Source: CAD feature listing. Evaluate the final solid. Frame: model axes, mm. A direction names the side the tool comes from. Give positions to 0.01 mm unless a question says otherwise; leave off trailing zeros. Answer in a Markdown table with one row per item.
```python
from build123d import *

# Parameters (mm, degrees)
SKETCH1_R            = 150
BOSS_EXTRUDE3_DEPTH  = 10
CUT_EXTRUDE2_DEPTH   = 10
BOSS_EXTRUDE4_DEPTH  = 1.8
SKETCH6_W            = 3
SKETCH6_H            = 7
BOSS_EXTRUDE5_DEPTH  = 2
SKETCH7_W            = 7
SKETCH7_H            = 3
BOSS_EXTRUDE6_DEPTH  = 2
SKETCH8_W            = 10
SKETCH8_H            = 10
CUT_EXTRUDE3_DEPTH   = 5
SKETCH9_W            = 9.193751657
SKETCH9_H            = 8.277315045
BOSS_EXTRUDE7_DEPTH  = 4.35
CHAMFER1_SIZE        = 1
CUT_EXTRUDE4_DEPTH   = 1.7
CUT_EXTRUDE5_DEPTH   = 0.8
FILLET1_R            = 3
FILLET2_R            = 1.4
SKETCH12_W           = 10.671911796
SKETCH12_H           = 9.690192172
CUT_EXTRUDE6_DEPTH   = 11
SKETCH13_W           = 9.731136712
SKETCH13_H           = 8.6
BOSS_EXTRUDE8_DEPTH  = 10
SKETCH14_W           = 9.731136712
SKETCH14_H           = 8.6
CUT_EXTRUDE7_DEPTH   = 5
FILLET3_R            = 1
FILLET4_R            = 1.2
CUT_EXTRUDE8_DEPTH   = 3.5
FILLET5_R            = 2.5
FILLET6_R            = 9
SKETCH16_W           = 0.25
SKETCH16_H           = 5
BOSS_EXTRUDE9_DEPTH  = 11.5
SKETCH17_W           = 9.5
SKETCH17_H           = 5
BOSS_EXTRUDE12_DEPTH = 0.13
SKETCH19_W           = 9.5
SKETCH19_H           = 5
BOSS_EXTRUDE13_DEPTH = 0.85
CHAMFER2_SIZE        = 1


with BuildPart() as part:
    # Sketch1 → Boss-Extrude3 (new body)
    with BuildSketch(Plane(origin=(0, 0, 0), x_dir=(1, 0, 0), z_dir=(0, 1, 0))):
        with Locations(Location((0, 0, 0), (0, 0, 270))):
            Circle(SKETCH1_R)
    extrude(amount=BOSS_EXTRUDE3_DEPTH)

    # Sketch4 → Cut-Extrude2 (cut)
    with BuildSketch(Plane(origin=(0, 10, 0), x_dir=(1, 0, 0), z_dir=(0, 1, 0))):
        Polygon((0, 0), (0, 162.329653064), (183.678217859, 162.329653064), (183.678217859, -176.427761891), (-217.916482153, -176.427761891), (-217.916482153, 0), align=None)
    extrude(amount=-CUT_EXTRUDE2_DEPTH, mode=Mode.SUBTRACT)

    # Sketch5 → Boss-Extrude4 (add)
    with BuildSketch(Plane(origin=(0, 10, 0), x_dir=(1, 0, 0), z_dir=(0, 1, 0))):
        with BuildLine():
            Line((0, 3.825), (0, 0))
            Line((0, 0), (-3.825, 0))
            ThreePointArc((-3.825, 0), (-2.704683438, 2.704683438), (0, 3.825))
        make_face()
    extrude(amount=BOSS_EXTRUDE4_DEPTH)

    # Sketch6 → Boss-Extrude5 (add)
    with BuildSketch(Plane(origin=(0, 10, 0), x_dir=(1, 0, 0), z_dir=(0, 1, 0))):
        with Locations((-28.5, 3.5)):
            Rectangle(SKETCH6_W, SKETCH6_H)
    extrude(amount=BOSS_EXTRUDE5_DEPTH)

    # Sketch7 → Boss-Extrude6 (add)
    with BuildSketch(Plane(origin=(0, 10, 0), x_dir=(1, 0, 0), z_dir=(0, 1, 0))):
        with Locations((-3.5, 28.5)):
            Rectangle(SKETCH7_W, SKETCH7_H)
    extrude(amount=BOSS_EXTRUDE6_DEPTH)

    # Sketch8 → Cut-Extrude3 (cut)
    with BuildSketch(Plane(origin=(0, 10, 0), x_dir=(1, 0, 0), z_dir=(0, 1, 0))):
        with Locations((-95, 5)):
            Rectangle(SKETCH8_W, SKETCH8_H)
    extrude(amount=-CUT_EXTRUDE3_DEPTH, mode=Mode.SUBTRACT)

    # Sketch9 → Boss-Extrude7 (add)
    with BuildSketch(Plane(origin=(0, 10, 0), x_dir=(1, 0, 0), z_dir=(0, 1, 0))):
        with Locations((4.596875828, 95.138657523)):
            Rectangle(SKETCH9_W, SKETCH9_H)
    extrude(amount=-BOSS_EXTRUDE7_DEPTH)

    # Chamfer1
    chamfer1_edges = [part.edges().sort_by_distance(p)[0] for p in [
        (9.193751657, 7.825, -99.277315045),
        (9.193751657, 7.825, -91),
    ]]
    chamfer(chamfer1_edges, length=CHAMFER1_SIZE)

    # Sketch10 → Cut-Extrude4 (cut)
    with BuildSketch(Plane.XZ):
        with BuildLine():
            Line((-140.926536809, 0), (-144.178447036, 0))
            ThreePointArc((-144.178447036, 0), (-101.9495576, -101.9495576), (0, -144.178447036))
            Line((0, -144.178447036), (0, -140.926536809))
            ThreePointArc((0, -140.926536809), (-99.650109827, -99.650109827), (-140.926536809, 0))
        make_face()
    extrude(amount=-CUT_EXTRUDE4_DEPTH, mode=Mode.SUBTRACT)

    # Sketch11 → Cut-Extrude5 (cut)
    with BuildSketch(Plane(origin=(0, 0, 0), x_dir=(-1, 0, 0), z_dir=(0, -1, 0))):
        Polygon((47, 0), (50, 0), (50, 50), (0, 50), (0, 47), (47, 47), align=None)
    extrude(amount=-CUT_EXTRUDE5_DEPTH, mode=Mode.SUBTRACT)

    # Fillet1
    fillet1_edges = [part.edges().sort_by_distance(p)[0] for p in [
        (-106.066017178, 0, -106.066017178),
    ]]
    fillet(fillet1_edges, radius=FILLET1_R)

    # Fillet2
    fillet2_edges = [part.edges().sort_by_distance(p)[0] for p in [
        (0, 5.65, -95.138657523),
    ]]
    fillet(fillet2_edges, radius=FILLET2_R)

    # Sketch12 → Cut-Extrude6 (cut)
    with BuildSketch(Plane(origin=(0, 0, 0), x_dir=(-1, 0, 0), z_dir=(0, -1, 0))):
        with Locations((-5.335955898, 95.265421493)):
            Rectangle(SKETCH12_W, SKETCH12_H)
    extrude(amount=-CUT_EXTRUDE6_DEPTH, mode=Mode.SUBTRACT)

    # Sketch13 → Boss-Extrude8 (add)
    with BuildSketch(Plane(origin=(0, 0, 0), x_dir=(-1, 0, 0), z_dir=(0, -1, 0))):
        with Locations((-4.865568356, 95.8)):
            Rectangle(SKETCH13_W, SKETCH13_H)
    extrude(amount=-BOSS_EXTRUDE8_DEPTH)

    # Sketch14 → Cut-Extrude7 (cut)
    with BuildSketch(Plane(origin=(0, 0, 0), x_dir=(-1, 0, 0), z_dir=(0, -1, 0))):
        with Locations((-4.865568356, 95.8)):
            Rectangle(SKETCH14_W, SKETCH14_H)
    extrude(amount=-CUT_EXTRUDE7_DEPTH, mode=Mode.SUBTRACT)

    # Fillet3
    fillet3_edges = [part.edges().sort_by_distance(p)[0] for p in [
        (0, 5, -95.8),
    ]]
    fillet(fillet3_edges, radius=FILLET3_R)

    # Fillet4
    fillet4_edges = [part.edges().sort_by_distance(p)[0] for p in [
        (9.731136712, 7.5, -91.5),
        (9.731136712, 7.5, -100.1),
    ]]
    fillet(fillet4_edges, radius=FILLET4_R)

    # Sketch15 → Cut-Extrude8 (cut)
    with BuildSketch(Plane(origin=(0, 10, 0), x_dir=(1, 0, 0), z_dir=(0, 1, 0))):
        with BuildLine():
            Line((-84.010224854, 7.071067812), (-84.010224854, 17.341351392))
            Line((-84.010224854, 17.341351392), (-106.385767568, 17.341351392))
            Line((-106.385767568, 17.341351392), (-106.385767568, 7.071067812))
            Line((-106.385767568, 7.071067812), (-139.141411083, 7.071067812))
            ThreePointArc((-139.141411083, 7.071067812), (-98.514801625, 98.514801625), (-7.071067812, 139.141411083))
            Line((-7.071067812, 139.141411083), (-7.071067812, 59.581876439))
            ThreePointArc((-7.071067812, 59.581876439), (-42.426406871, 42.426406871), (-59.581876439, 7.071067812))
            Line((-59.581876439, 7.071067812), (-84.010224854, 7.071067812))
        make_face()
    extrude(amount=-CUT_EXTRUDE8_DEPTH, mode=Mode.SUBTRACT)

    # Fillet5
    fillet5_edges = [part.edges().sort_by_distance(p)[0] for p in [
        (-84.010224854, 8.25, -17.341351392),
        (-106.385767568, 8.25, -17.341351392),
    ]]
    fillet(fillet5_edges, radius=FILLET5_R)

    # Fillet6
    # the kernel refuses this fillet: 9 mm, written as the material it adds along each edge
    with BuildSketch(Plane(origin=(-103.885767568, 6.5, -14.841351392), x_dir=(-1, 0, 0), z_dir=(0, 0, 1))) as fillet6_piece_1:
        with BuildLine():
            CenterArc((9.623903424, -9), FILLET6_R, 90, 52.330113036)
            Line((9.623903424, 0), (2.5, 0))
            Line((2.5, 0), (2.5, -3.5))
        make_face()
    revolve(axis=Axis((-103.885767568, 6.5, -14.841351392), (0, -1, 0)), revolution_arc=90)
    with BuildSketch(Plane(origin=(-86.510224854, 6.5, -14.841351392), x_dir=(0, 0, -1), z_dir=(-1, 0, 0))) as fillet6_piece_2:
        with BuildLine():
            CenterArc((9.623903424, -9), FILLET6_R, 90, 52.330113036)
            Line((9.623903424, 0), (2.5, 0))
            Line((2.5, 0), (2.5, -3.5))
        make_face()
    revolve(axis=Axis((-86.510224854, 6.5, -14.841351392), (0, -1, 0)), revolution_arc=90)
    with BuildSketch(Plane(origin=(0, 6.5, 0), x_dir=(-0.9970291212395074, 0, 0.07702552434340171), z_dir=(0.07702552434340171, 0, 0.9970291212395074))) as fillet6_piece_3_section:
        with BuildLine():
            CenterArc((132.197065128, -9), FILLET6_R, 37.669886964, 52.330113036)
            Line((132.197065128, 0), (139.320968552, 0))
            Line((139.320968552, 0), (139.320968552, -3.5))
        make_face()
    fillet6_piece_3 = revolve(axis=Axis((0, 6.5, 0), (0, -1, 0)), revolution_arc=98.835226115, mode=Mode.PRIVATE)
    fillet6_piece_3 = split(fillet6_piece_3, bisect_by=Plane(origin=(0, 6.5, 0), z_dir=(-1, 0, 0)), keep=Keep.TOP, mode=Mode.PRIVATE)
    fillet6_piece_3 = split(fillet6_piece_3, bisect_by=Plane(origin=(0, 6.5, 0), z_dir=(0, 0, -1)), keep=Keep.TOP, mode=Mode.PRIVATE)
    add(fillet6_piece_3)
    with BuildSketch(Plane(origin=(-88.576009007, 6.5, -7.071067812), x_dir=(0, 1, 0), z_dir=(-1, 0, 0))) as fillet6_piece_4_section:
        with BuildLine():
            CenterArc((9, 7.123903424), FILLET6_R, 180, 52.330113036)
            Line((0, 7.123903424), (0, 0))
            Line((0, 0), (3.5, 0))
        make_face()
    fillet6_piece_4 = extrude(amount=68.375160637, mode=Mode.PRIVATE)
    fillet6_piece_4 = fillet6_piece_4 & Plane(origin=(0, 6.5, 0), x_dir=(0, 0, 1), z_dir=(0, -1, 0)) * Cylinder(150, 166, mode=Mode.PRIVATE)
    fillet6_piece_4 = split(fillet6_piece_4, bisect_by=Plane(origin=(-100, 6.5, -7.071067812), z_dir=(-1, 0, 0)), keep=Keep.TOP, mode=Mode.PRIVATE)
    add(fillet6_piece_4)
    with BuildSketch(Plane(origin=(-86.510224854, 6.5, -17.341351392), x_dir=(0, 1, 0), z_dir=(-1, 0, 0))) as fillet6_piece_5:
        with BuildLine():
            CenterArc((9, 7.123903424), FILLET6_R, 180, 52.330113036)
            Line((0, 7.123903424), (0, 0))
            Line((0, 0), (3.5, 0))
        make_face()
    extrude(amount=17.375542715)
    with BuildSketch(Plane(origin=(-41.772117878, 6.5, -7.071067812), x_dir=(0, 1, 0), z_dir=(-1, 0, 0))) as fillet6_piece_6_section:
        with BuildLine():
            CenterArc((9, 7.123903424), FILLET6_R, 180, 52.330113036)
            Line((0, 7.123903424), (0, 0))
            Line((0, 0), (3.5, 0))
        make_face()
    fillet6_piece_6 = extrude(amount=60.047865536, mode=Mode.PRIVATE)
    fillet6_piece_6 = split(fillet6_piece_6, bisect_by=Plane(origin=(-90, 6.5, -7.071067812), z_dir=(1, 0, 0)), keep=Keep.TOP, mode=Mode.PRIVATE)
    add(fillet6_piece_6)
    with BuildSketch(Plane(origin=(-7.071067812, 6.5, -156.951169644), x_dir=(0, 1, 0), z_dir=(0, 0, 1))) as fillet6_piece_7_section:
        with BuildLine():
            CenterArc((9, 7.123903424), FILLET6_R, 180, 52.330113036)
            Line((0, 7.123903424), (0, 0))
            Line((0, 0), (3.5, 0))
        make_face()
    fillet6_piece_7 = extrude(amount=115.179051766, mode=Mode.PRIVATE)
    fillet6_piece_7 = fillet6_piece_7 & Plane(origin=(0, 6.5, 0), x_dir=(0, 0, 1), z_dir=(0, -1, 0)) * Cylinder(150, 259, mode=Mode.PRIVATE)
    add(fillet6_piece_7)
    with BuildSketch(Plane(origin=(0, 6.5, 0), x_dir=(0.17783871438849583, 0, -0.9840596484282074), z_dir=(0.9840596484282074, 0, 0.17783871438849583))) as fillet6_piece_8_section:
        with BuildLine():
            CenterArc((67.123903424, 9), FILLET6_R, 217.669886964, 52.330113036)
            Line((67.123903424, 0), (60, 0))
            Line((60, 0), (60, 3.5))
        make_face()
    fillet6_piece_8 = revolve(axis=Axis((0, 6.5, 0), (0, 1, 0)), revolution_arc=110.487792536, mode=Mode.PRIVATE)
    fillet6_piece_8 = split(fillet6_piece_8, bisect_by=Plane(origin=(0, 6.5, 0), z_dir=(-1, 0, 0)), keep=Keep.TOP, mode=Mode.PRIVATE)
    fillet6_piece_8 = split(fillet6_piece_8, bisect_by=Plane(origin=(0, 6.5, 0), z_dir=(0, 0, -1)), keep=Keep.TOP, mode=Mode.PRIVATE)
    add(fillet6_piece_8)
    with BuildSketch(Plane(origin=(-84.010224854, 6.5, 10.738690749), x_dir=(0, 1, 0), z_dir=(0, 0, -1))) as fillet6_piece_9_section:
        with BuildLine():
            CenterArc((9, 7.123903424), FILLET6_R, 180, 52.330113036)
            Line((0, 7.123903424), (0, 0))
            Line((0, 0), (3.5, 0))
        make_face()
    fillet6_piece_9 = extrude(amount=25.580042141, mode=Mode.PRIVATE)
    fillet6_piece_9 = split(fillet6_piece_9, bisect_by=Plane(origin=(-84.010224854, 6.5, 0), z_dir=(0, 0, -1)), keep=Keep.TOP, mode=Mode.PRIVATE)
    add(fillet6_piece_9)
    with BuildSketch(Plane(origin=(-106.385767568, 6.5, -14.841351392), x_dir=(0, 1, 0), z_dir=(0, 0, 1))) as fillet6_piece_10_section:
        with BuildLine():
            CenterArc((9, 7.123903424), FILLET6_R, 180, 52.330113036)
            Line((0, 7.123903424), (0, 0))
            Line((0, 0), (3.5, 0))
        make_face()
    fillet6_piece_10 = extrude(amount=25.580042141, mode=Mode.PRIVATE)
    fillet6_piece_10 = split(fillet6_piece_10, bisect_by=Plane(origin=(-106.385767568, 6.5, 0), z_dir=(0, 0, -1)), keep=Keep.TOP, mode=Mode.PRIVATE)
    add(fillet6_piece_10)

    # Sketch16 → Boss-Extrude9 (add)
    with BuildSketch(Plane.XY):
        with Locations((-99.875, 7.5)):
            Rectangle(SKETCH16_W, SKETCH16_H)
        with Locations((-90.125, 7.5)):
            Rectangle(SKETCH16_W, SKETCH16_H)
    extrude(amount=-BOSS_EXTRUDE9_DEPTH)

    # Sketch17 → Boss-Extrude12 (add)
    with BuildSketch(Plane.XY.offset(-10)):
        with Locations((-95, 7.5)):
            Rectangle(SKETCH17_W, SKETCH17_H)
    extrude(amount=BOSS_EXTRUDE12_DEPTH)

    # Sketch19 → Boss-Extrude13 (add)
    with BuildSketch(Plane.XY.offset(-9.87)):
        with Locations((-95, 7.5)):
            Rectangle(SKETCH19_W, SKETCH19_H)
    extrude(amount=BOSS_EXTRUDE13_DEPTH)

    # Chamfer2
    chamfer2_edges = [part.edges().sort_by_distance(p)[0] for p in [
        (-99.75, 7.5, 0),
        (-90.25, 7.5, 0),
    ]]
    chamfer(chamfer2_edges, length=CHAMFER2_SIZE)


solid = part.part
```
1) Pull-direction query (X, two-part tool) for faces 5 (the cylindrical face through (-107.23, 6.45, -104.89)), 6 (the cylindrical face through (-95.076, 7.397, -20.548)), 7 (the flat face through (-76, 5, 0)), 8 (the cylindrical face through (-2.734, 10.887, -2.675)); classes: released by +X, released by -X, zero draft, split by the parting line, or undercut.
Reply:
| item | result |
|---|---|
| face 5 | released by -X |
| face 6 | undercut |
| face 7 | zero draft |
| face 8 | undercut |
2) Pin query (flat end, axial travel): pin 1 Ø0.6 at (x, y) = (-14.5, 0.5) entering from -Z; pin 2 Ø1.8 at (x, y) = (3, 7) entering from -Z; pin 3 Ø5.5 at (y, z) = (7, -6.5) entering from +X. Return the tip coordinate at first contact, or that it passes through.
Reply:
| item | result |
|---|---|
| pin 1 | stops at z = -148.33 |
| pin 2 | stops at z = -100.1 |
| pin 3 | stops at x = 0 |
3) Set-up query: faces 1 (the flat face through (-95, 8, -9.02)), 2 (the cylindrical face through (-98.55, 0.84, -100.74)), 3 (the cylindrical face through (-71.625, 7.836, -9.477)), 4 (the flat face through (4, 8, -100.1)). Return all of +Z, -Z, +X, -X, +Y, -Y with unobstructed straight access to the full face (end or side cutting, diameter ignored); none if empty.
Reply:
| item | result |
|---|---|
| face 1 | +Z, +Y |
| face 2 | -Y |
| face 3 | +Y |
| face 4 | -Z, +X, +Y, -Y |
4) Material intervals for L1, parallel to Y at x = -24.5, z = -39; L2, parallel to Y at x = -78, z = -83; L3, parallel to X at y = 7, z = -8, sorted ascending.
Reply:
| item | result |
|---|---|
| L1 | y = 0 to 10 |
| L2 | y = 0 to 6.5 |
| L3 | x = -149.79 to -99.75, -90.25 to 0 |
